```python
from build123d import *

# Parameters (mm, degrees)
F1_DEPTH = 5
F2_R     = 2
F3_R     = 3.5
F4_R     = 1.5


with BuildPart() as f1:
    # F0 (on Top) → F1 (new body)
    with BuildSketch(Plane.XY):
        with BuildLine():
            Line((-17.3243107274, 26.09127976), (-17.3243107274, -23.90872024))
            ThreePointArc((-17.3243107274, -23.90872024), (-15.8598446334, -27.4442541459), (-12.3243107274, -28.90872024))
            Line((-12.3243107274, -28.90872024), (-3.8243107274, -28.90872024))
            Line((-3.8243107274, -28.90872024), (-3.8243107274, -24.65872024))
            ThreePointArc((-3.8243107274, -24.65872024), (-5.5743107274, -22.90872024), (-3.8243107274, -21.15872024))
            Line((-3.8243107274, -21.15872024), (-3.8243107274, -12.45872024))
            Line((-3.8243107274, -12.45872024), (-5.4945183623, -12.45872024))
            ThreePointArc((-5.4945183623, -12.45872024), (-5.8691381363, -12.3035476489), (-6.0243107274, -11.9289278748))
            Line((-6.0243107274, -11.9289278748), (-6.0243107274, -6.6885126051))
            ThreePointArc((-6.0243107274, -6.6885126051), (-5.8691381363, -6.3138928311), (-5.4945183623, -6.15872024))
            Line((-5.4945183623, -6.15872024), (-3.8243107274, -6.15872024))
            Line((-3.8243107274, -6.15872024), (-3.8243107274, -2.15872024))
            ThreePointArc((-3.8243107274, -2.15872024), (-7.0743107274, 1.09127976), (-3.8243107274, 4.34127976))
            Line((-3.8243107274, 4.34127976), (-3.8243107274, 8.34127976))
            Line((-3.8243107274, 8.34127976), (-5.4945183623, 8.34127976))
            ThreePointArc((-5.4945183623, 8.34127976), (-5.8691381363, 8.4964523511), (-6.0243107274, 8.8710721252))
            Line((-6.0243107274, 8.8710721252), (-6.0243107274, 14.1114873949))
            ThreePointArc((-6.0243107274, 14.1114873949), (-5.8691381363, 14.4861071689), (-5.4945183623, 14.64127976))
            Line((-5.4945183623, 14.64127976), (-3.8243107274, 14.64127976))
            Line((-3.8243107274, 14.64127976), (-3.8243107274, 23.34127976))
            ThreePointArc((-3.8243107274, 23.34127976), (-5.5743107274, 25.09127976), (-3.8243107274, 26.84127976))
            Line((-3.8243107274, 26.84127976), (-3.8243107274, 31.09127976))
            Line((-3.8243107274, 31.09127976), (-12.3243107274, 31.09127976))
            ThreePointArc((-12.3243107274, 31.09127976), (-15.8598446334, 29.6268136659), (-17.3243107274, 26.09127976))
        make_face()
        with BuildLine():
            Line((-3.8243107274, -24.65872024), (-3.8243107274, -28.90872024))
            Line((-3.8243107274, -28.90872024), (4.6756892726, -28.90872024))
            ThreePointArc((4.6756892726, -28.90872024), (8.2112231785, -27.4442541459), (9.6756892726, -23.90872024))
            Line((9.6756892726, -23.90872024), (9.6756892726, 0))
            Line((9.6756892726, 0), (-0.584877345, 0.8294184204))
            ThreePointArc((-0.584877345, 0.8294184204), (-1.6207396886, -1.2976058959), (-3.8243107274, -2.15872024))
            Line((-3.8243107274, -2.15872024), (-3.8243107274, -6.15872024))
            Line((-3.8243107274, -6.15872024), (-2.1541030926, -6.15872024))
            ThreePointArc((-2.1541030926, -6.15872024), (-1.7794833185, -6.3138928311), (-1.6243107274, -6.6885126051))
            Line((-1.6243107274, -6.6885126051), (-1.6243107274, -11.9289278748))
            ThreePointArc((-1.6243107274, -11.9289278748), (-1.7794833185, -12.3035476489), (-2.1541030926, -12.45872024))
            Line((-2.1541030926, -12.45872024), (-3.8243107274, -12.45872024))
            Line((-3.8243107274, -12.45872024), (-3.8243107274, -21.15872024))
            ThreePointArc((-3.8243107274, -21.15872024), (-2.5868738603, -21.6712833729), (-2.0743107274, -22.90872024))
            ThreePointArc((-2.0743107274, -22.90872024), (-2.5868738603, -24.1461571071), (-3.8243107274, -24.65872024))
        make_face()
        with BuildLine():
            Line((4.6756892726, 31.09127976), (-3.8243107274, 31.09127976))
            Line((-3.8243107274, 31.09127976), (-3.8243107274, 26.84127976))
            ThreePointArc((-3.8243107274, 26.84127976), (-2.5868738603, 26.3287166271), (-2.0743107274, 25.09127976))
            ThreePointArc((-2.0743107274, 25.09127976), (-2.5868738603, 23.8538428929), (-3.8243107274, 23.34127976))
            Line((-3.8243107274, 23.34127976), (-3.8243107274, 14.64127976))
            Line((-3.8243107274, 14.64127976), (-2.1541030926, 14.64127976))
            ThreePointArc((-2.1541030926, 14.64127976), (-1.7794833185, 14.4861071689), (-1.6243107274, 14.1114873949))
            Line((-1.6243107274, 14.1114873949), (-1.6243107274, 8.8710721252))
            ThreePointArc((-1.6243107274, 8.8710721252), (-1.7794833185, 8.4964523511), (-2.1541030926, 8.34127976))
            Line((-2.1541030926, 8.34127976), (-3.8243107274, 8.34127976))
            Line((-3.8243107274, 8.34127976), (-3.8243107274, 4.34127976))
            ThreePointArc((-3.8243107274, 4.34127976), (-1.5262136886, 3.3893767989), (-0.5743107274, 1.09127976))
            ThreePointArc((-0.5743107274, 1.09127976), (-0.5769534563, 0.9602425377), (-0.584877345, 0.8294184204))
            Line((-0.584877345, 0.8294184204), (9.6756892726, 0))
            Line((9.6756892726, 0), (9.6756892726, 26.09127976))
            ThreePointArc((9.6756892726, 26.09127976), (8.2112231785, 29.6268136659), (4.6756892726, 31.09127976))
        make_face()
    extrude(amount=F1_DEPTH)

    # F2
    f2_edges = [f1.edges().sort_by_distance(p)[0] for p in [
        (-3.824311, -24.65872, 5),
        (-3.824311, 23.34128, 5),
    ]]
    fillet(f2_edges, radius=F2_R)

    # F3
    f3_edges = [f1.edges().sort_by_distance(p)[0] for p in [
        (-3.824311, -2.15872, 0),
    ]]
    fillet(f3_edges, radius=F3_R)

    # F4
    f4_edges = [f1.edges().sort_by_distance(p)[0] for p in [
        (-17.324311, 1.09128, 5),
    ]]
    fillet(f4_edges, radius=F4_R)


solid = f1.part
```
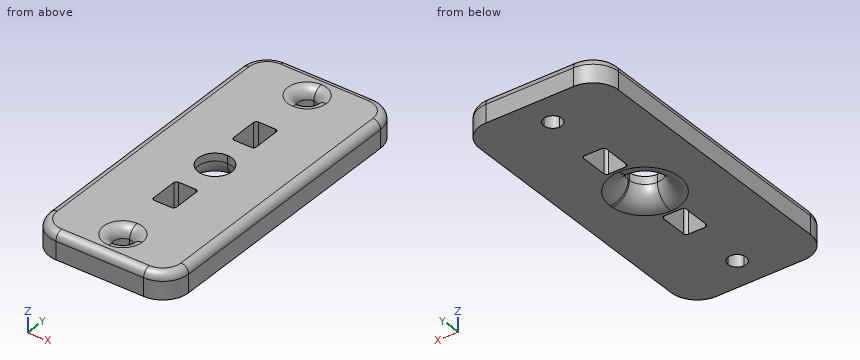
Can you work these out from the model? Positions are in its coordinate system, mm. Give positions to 0.01 mm unless a question says otherwise; leave off trailing zeros. Order: outer loops, then holes, each group sorted by start corner. A loop starts at its lowest first (then second) coordinate and runs counter-clockwise, first axis right, second up. Notation, with made-up numbers: M 6,35.5 L 60,35.5 A25 cw 60,62.5 Z; hole C 84.5,62.25 d7. An arc over 180 degrees is marked long. Write item = value, one per line. Start each with the question number.
Q1. Suppose I cut it at A-A (y = 12.5). Write out the boundary of the cut face in (x, z), plus the area to 3 significant figures.
Q2. Suppose I cut it at B-B (z = 1.3). Write out the boundary of the cut face in (x, y).
Q3. Suppose I cut it at C-C (z = 4.2). Write out the boundary of the cut face in (x, y).
Q4. I need wall thicknesses on probe 1 along X at (y, z) = (14, 2.1); probe 2 along Y at (x, z) = (-2.75, 0.95); probe 3 along Y at (x, z) = (-4, 3.5). Which ranges of each line are inside material? Lowest first, please. Write a range as [from, to].
Q5. Will this pin go through, and if not, where does the flat tip stop? pin 1 Ø2 at (x, y) = (-7, -15) entering from -Z.
Check result:
q1.outline = M -17.32,0 L -6.02,0 L -6.02,5 L -15.82,5 A1.5 ccw -17.32,3.5 Z; M -1.62,0 L 9.68,0 L 9.68,3.5 A1.5 ccw 8.18,5 L -1.62,5 Z
q1.area = 112 mm2
q2.outline = M -17.32,-23.91 A5 ccw -12.32,-28.91 L 4.68,-28.91 A5 ccw 9.68,-23.91 L 9.68,26.09 A5 ccw 4.68,31.09 L -12.32,31.09 A5 ccw -17.32,26.09 Z; hole C -3.82,1.09 d8.06; hole M -6.02,-11.93 A0.53 ccw -5.49,-12.46 L -2.15,-12.46 A0.53 ccw -1.62,-11.93 L -1.62,-6.69 A0.53 ccw -2.15,-6.16 L -5.49,-6.16 A0.53 ccw -6.02,-6.69 Z; hole M -6.02,8.87 A0.53 ccw -5.49,8.34 L -2.15,8.34 A0.53 ccw -1.62,8.87 L -1.62,14.11 A0.53 ccw -2.15,14.64 L -5.49,14.64 A0.53 ccw -6.02,14.11 Z; hole C -3.82,-22.91 d3.5; hole C -3.82,25.09 d3.5
q3.outline = M -17.15,-23.91 A4.83 ccw -12.32,-28.74 L 4.68,-28.74 A4.83 ccw 9.5,-23.91 L 9.5,26.09 A4.83 ccw 4.68,30.92 L -12.32,30.92 A4.83 ccw -17.15,26.09 Z; hole C -3.82,1.09 d6.5; hole M -6.02,-11.93 A0.53 ccw -5.49,-12.46 L -2.15,-12.46 A0.53 ccw -1.62,-11.93 L -1.62,-6.69 A0.53 ccw -2.15,-6.16 L -5.49,-6.16 A0.53 ccw -6.02,-6.69 Z; hole M -6.02,8.87 A0.53 ccw -5.49,8.34 L -2.15,8.34 A0.53 ccw -1.62,8.87 L -1.62,14.11 A0.53 ccw -2.15,14.64 L -5.49,14.64 A0.53 ccw -6.02,14.11 Z; hole C -3.82,-22.91 d4.3; hole C -3.82,25.09 d4.3
q4.probe_1 = [-17.32, -6.02], [-1.62, 9.68]
q4.probe_2 = [-28.91, -24.29], [-21.53, -12.46], [-6.16, -3.13], [5.31, 8.34], [14.64, 23.71], [26.47, 31.09]
q4.probe_3 = [-28.91, -24.71], [-21.1, -12.46], [-6.16, -2.15], [4.34, 8.34], [14.64, 23.29], [26.9, 31.09]
q5.pin_1 = 0
